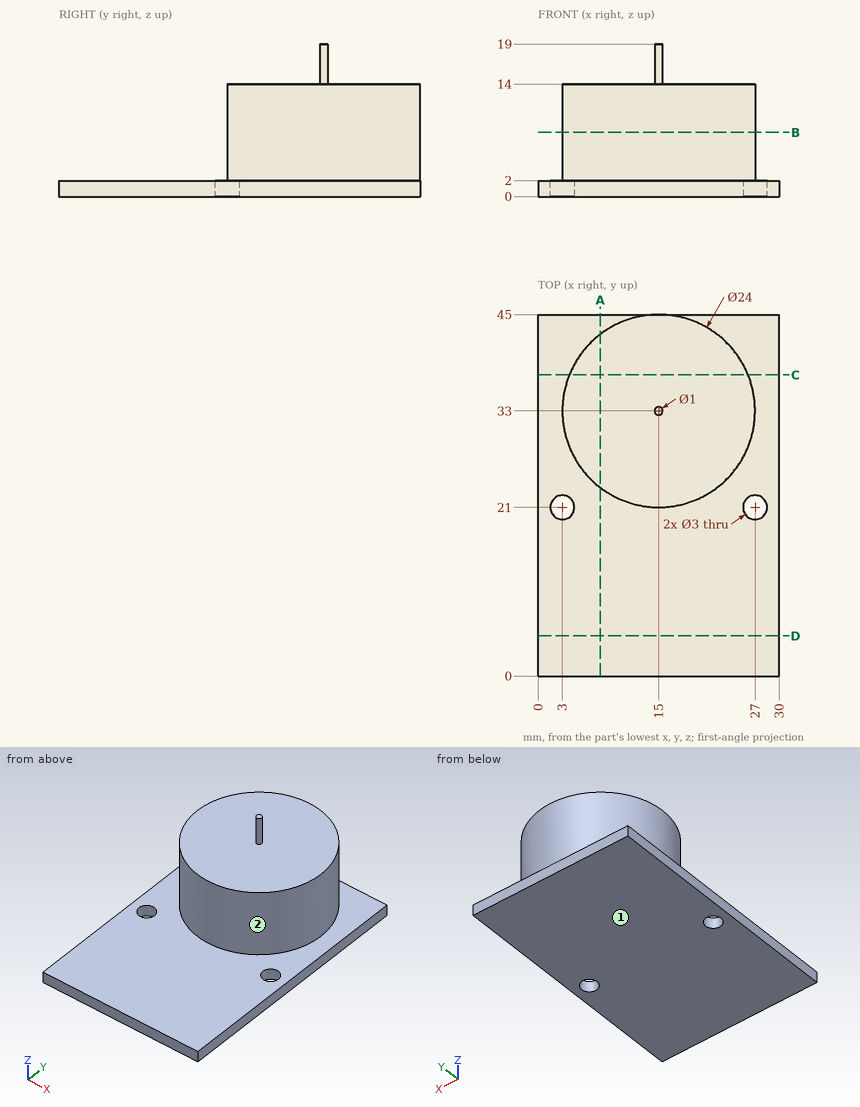
Check sheet for the drawn part. Datum: minimum x, y, z corner. Units: mm. A direction names the side the tool comes from. Round coordinates to 2 decimals unless told otherwise and drop trailing zeros. Loops run counter-clockwise (first coordinate to the right, second up) from the corner with the lowest first, then second, coordinate; pieces in that order, holes last.
Item 1: Cross-section at B-B on z = 8. Record the boundary of the cut face in (x, y), then the cut area to 3 significant figures.
Item 2: Cross-section at C-C on y = 37.5. Record the boundary of the cut face in (x, z), then the cut area to 3 significant figures.
Item 3: Cross-section at D-D on y = 5. Record the boundary of the cut face in (x, z).
Item 4: Gauge pin test, flat ends, axial feed: pin 1 (5 mm diameter, centred on x = 25.5, y = 7, fed in from +Z); pin 2 (12 mm diameter, centred on x = 6, y = 40.5, fed in from +Z); pin 3 (10 mm diameter, centred on x = 23, z = 10.5, fed in from +Y). Record the tip position at first contact, or that the pin passes through.
Item 5: Cross-section at A-A on x = 7.75. Record the boundary of the cut face in (y, z).
Item 6: Thickness scan on line 1 (X direction, y = 20, z = 1.5); line 2 (Y direction, x = 27, z = 1); line 3 (Z direction, x = 14, y = 35). Record the ranges inside material, lowest first.
Item 7: Access from +Z, -Z, +X, -X, +Y, -Y to the whole of each face (thin tool, end or side, straight path). Record for the marked faces 1 and 2.
Answer sheet:
1. outline: circle Ø24 at (15, 33)
1. area: 452 mm2
2. outline: (0, 0) - (30, 0) - (30, 2) - (26.12, 2) - (26.12, 14) - (3.88, 14) - (3.88, 2) - (0, 2) - close
2. area: 327 mm2
3. outline: (0, 0) - (30, 0) - (30, 2) - (0, 2) - close
4. pin 1: stops at z = 2
4. pin 2: stops at z = 14
4. pin 3: stops at y = 44.62
5. outline: (0, 0) - (45, 0) - (45, 2) - (42.56, 2) - (42.56, 14) - (23.44, 14) - (23.44, 2) - (0, 2) - close
6. line 1: x = 0 to 1.88, 4.12 to 25.88, 28.12 to 30
6. line 2: y = 0 to 19.5, 22.5 to 45
6. line 3: z = 0 to 14
7. face 1: -Z, +X, -X, +Y, -Y
7. face 2: +Z
